Geometry check sheet. Reference: drawing and pictorial views, mm from the part's lowest x, y, z. Coordinates: 2 decimals unless noted, no trailing zeros. Loops run counter-clockwise (first coordinate to the right, second up) from the corner with the lowest first, then second, coordinate; pieces in that order, holes last. Notation, with made-up numbers: (-32, -28.75) -> (0, -28.75) arc R33 cw to (0, 2.25) -> close; hole circle Ø6 at (-14, 79). An arc over 180 degrees is marked (long way). Answer as a JSON object with one key per item and string values.
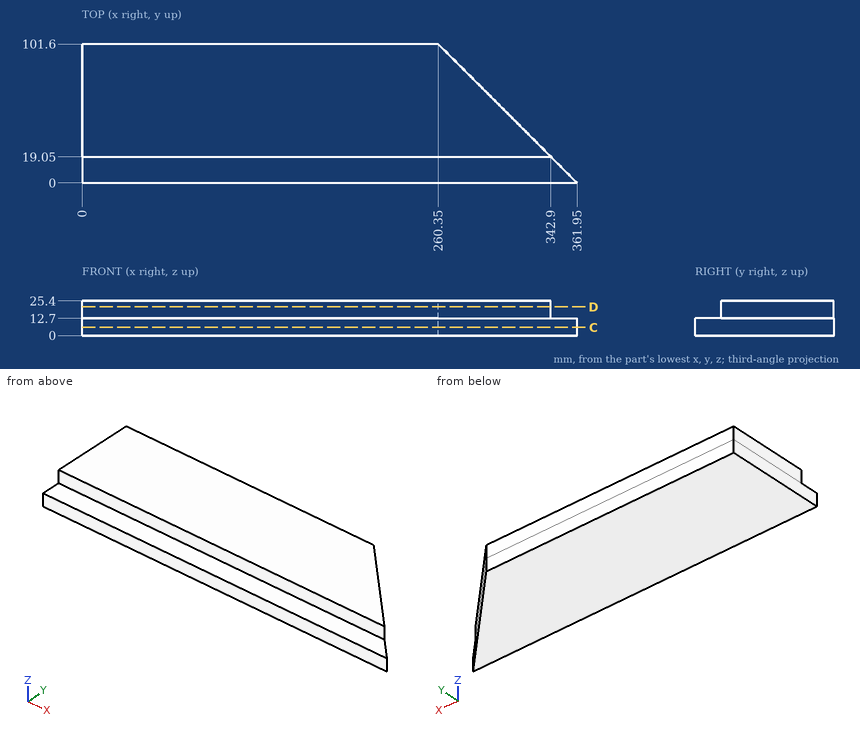
1. Section check C-C, the plane z = 6. Record the boundary of the cut face in (x, y), then the cut area to 3 significant figures.
Evaluation:
{"outline": "(0, 0) -> (361.95, 0) -> (260.35, 101.6) -> (0, 101.6) -> close", "area": "31,600 mm^2"}
2. Section check D-D, the plane z = 21. Record the boundary of the cut face in (x, y).
Evaluation:
{"outline": "(0, 19.05) -> (342.9, 19.05) -> (260.35, 101.6) -> (0, 101.6) -> close"}
3. Thickness scan on probe 1 along Y at (x, z) = (29.5, 14.5); probe 2 along Z at (x, y) = (63, 14); probe 3 along Y at (x, z) = (336.5, 15.25). Record the ranges inside material, lowest first. Write a range as from..to.
Evaluation:
{"probe 1": "y = 19.05..101.6", "probe 2": "z = 0..12.7", "probe 3": "y = 19.05..25.45"}
4. Depth check by flat-ended pin: P1, Ø10, axis at y = 79, z = 18.5, coming from the +X side; P2, Ø8, axis at y = 48.5, z = 2.5, coming from the +X side; P3, Ø12, axis at y = 47, z = 11, coming from the +X side. Enter the tip coordinate at first touch or a pass-through.
Evaluation:
{"P1": "stops at x = 287.95", "P2": "stops at x = 317.45", "P3": "stops at x = 320.95"}
